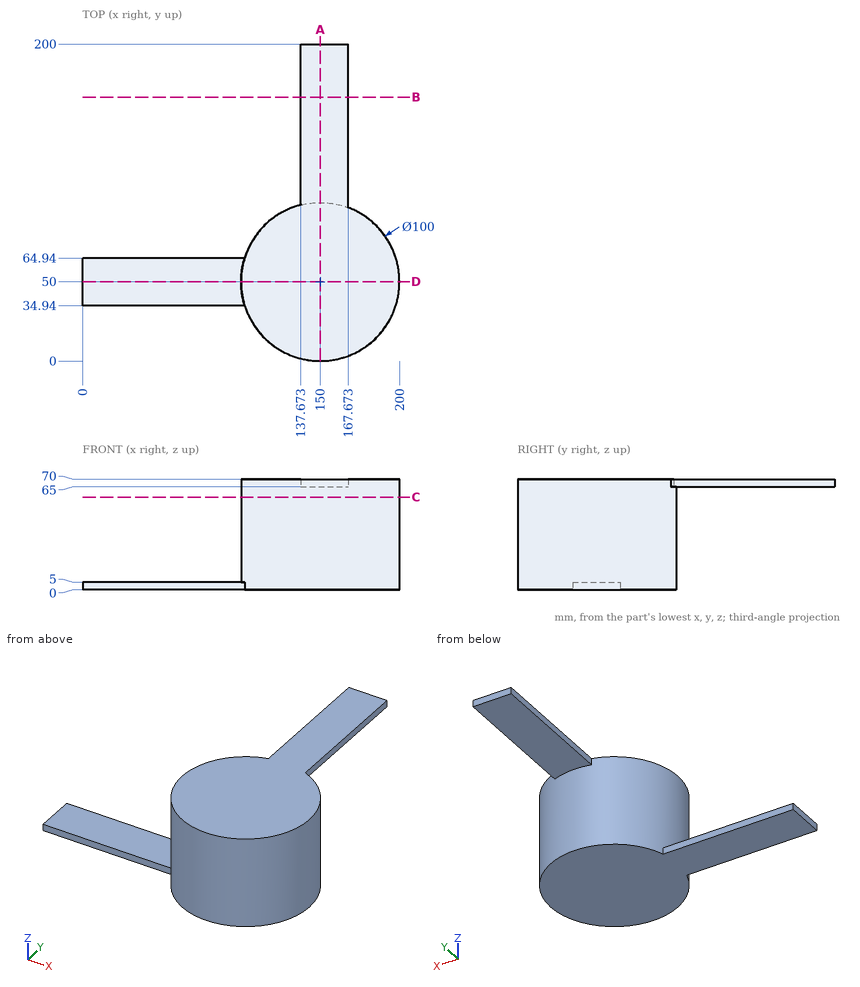
Part print with two shaded views. Sizes in mm from the minimum x, y, z corner. Coordinates: 2 decimals unless noted, no trailing zeros. Order: outer loops, then holes, each group sorted by start corner. A loop starts at its lowest first (then second) coordinate and runs counter-clockwise, first axis right, second up.
(1) Pin check, flat tips, straight feed: pin 1 Ø4 at (x, z) = (54, 2) entering from -Y; pin 2 Ø2.5 at (y, z) = (126, 67.5) entering from -X; pin 3 Ø4 at (y, z) = (171, 68) entering from +X. Stop position of each tip, or through.
Solution:
pin 1: stops at y = 34.94
pin 2: stops at x = 137.67
pin 3: stops at x = 167.67
(2) Drill centre lines: L1, parallel to Z at x = 57.5, y = 58.5; L2, parallel to Z at x = 161, y = 153; L3, parallel to Y at x = 151, z = 34. Where is each one in solid material? Low to high.
Solution:
L1: z = 0 to 5
L2: z = 65 to 70
L3: y = 0.01 to 99.99
(3) Saw through at C-C, the plane z = 58.5. Write the cut outline in (x, y), and give its area (3 significant figures).
Solution:
outline: circle Ø100 at (150, 50)
area: 7,850 mm2
(4) Saw through at D-D, the plane y = 50. Write the cut outline in (x, z), and give its area (3 significant figures).
Solution:
outline: (0, 0) - (200, 0) - (200, 70) - (100, 70) - (100, 5) - (0, 5) - close
area: 7,500 mm2
(5) Saw through at A-A, the plane x = 150. Write the cut outline in (y, z).
Solution:
outline: (0, 0) - (100, 0) - (100, 65) - (200, 65) - (200, 70) - (0, 70) - close
(6) Saw through at B-B, the plane y = 166.5. Write the cut outline in (x, z).
Solution:
outline: (137.67, 65) - (167.67, 65) - (167.67, 70) - (137.67, 70) - close
